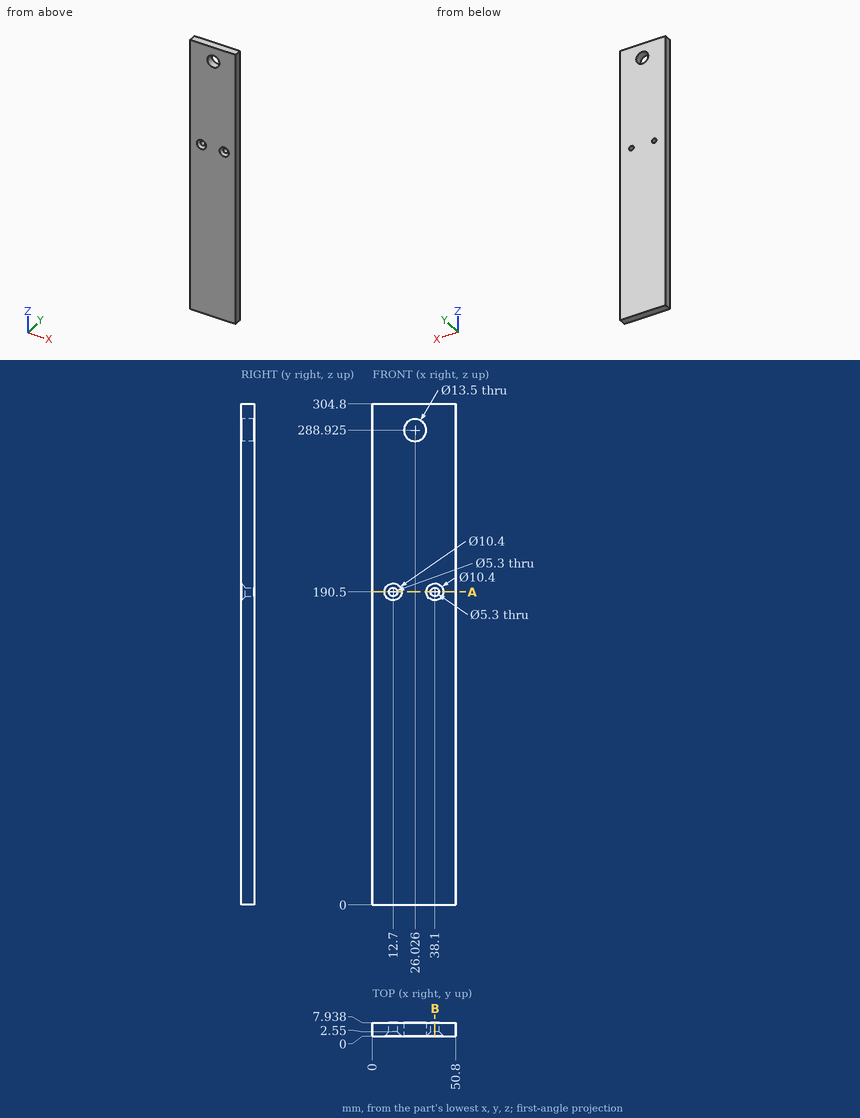
Geometry check sheet. Reference: drawing and pictorial views, mm from the part's lowest x, y, z. Give positions to 0.01 mm unless a question says otherwise; leave off trailing zeros. Order: outer loops, then holes, each group sorted by start corner. A loop starts at its lowest first (then second) coordinate and runs counter-clockwise, first axis right, second up. Notation, with made-up numbers: M 80,78.25 L 112,78.25 A29 ccw 112,102.25 Z; hole C 22.25,41 d2. An arc over 180 degrees is marked long. Answer in a Markdown table with one row per item. Add a question column.
Q1. Sectioned sample at B-B, the plane x = 38.1. Record the boundary of the cut face in (y, z).
Q2. Gauge pin test, flat ends, axial feed: pin 1 Ø2 at (x, y) = (18, 2) entering from -Z; pin 2 Ø8.5 at (x, z) = (12.7, 190.5) entering from -Y. Record the tip position at first contact, or that the pin passes through.
Q3. Sectioned sample at A-A, the plane z = 190.5. Record the boundary of the cut face in (x, y).
Q4. Thickness scan on L1, parallel to Z at x = 12.7, y = 5.5; L2, parallel to X at y = 6.75, z = 192 (1 decimal); L3, parallel to Z at x = 26, y = 6.75 (1 decimal). Record the ranges inside material, lowest first.
Verdict:
| question | item | result |
|---|---|---|
| 1 | outline | M 0,0 L 7.94,0 L 7.94,187.85 L 2.55,187.85 L 0,185.3 Z; M 0,195.7 L 2.55,193.15 L 7.94,193.15 L 7.94,304.8 L 0,304.8 Z |
| 2 | pin 1 | z = 0 |
| 2 | pin 2 | y = 0.95 |
| 3 | outline | M 0,0 L 7.5,0 L 10.05,2.55 L 10.05,7.94 L 0,7.94 Z; M 15.35,2.55 L 17.9,0 L 32.9,0 L 35.45,2.55 L 35.45,7.94 L 15.35,7.94 Z; M 40.75,2.55 L 43.3,0 L 50.8,0 L 50.8,7.94 L 40.75,7.94 Z |
| 4 | L1 | 0 to 187.85, 193.15 to 304.8 |
| 4 | L2 | 0 to 10.5, 14.9 to 35.9, 40.3 to 50.8 |
| 4 | L3 | 0 to 282.2, 295.7 to 304.8 |
